For this review, use the dimensioned drawing (mm, ordinates from the lowest corner) and the shaded views. A direction names the side the tool comes from. Coordinates: 2 decimals unless noted, no trailing zeros. Loops run counter-clockwise (first coordinate to the right, second up) from the corner with the lowest first, then second, coordinate; pieces in that order, holes last. Notation, with made-up numbers: M 88,72 L 109,72 A29 cw 109,107 Z; hole C 22,23.5 d2. An arc over 180 degrees is marked long. Write item = value, one per line.
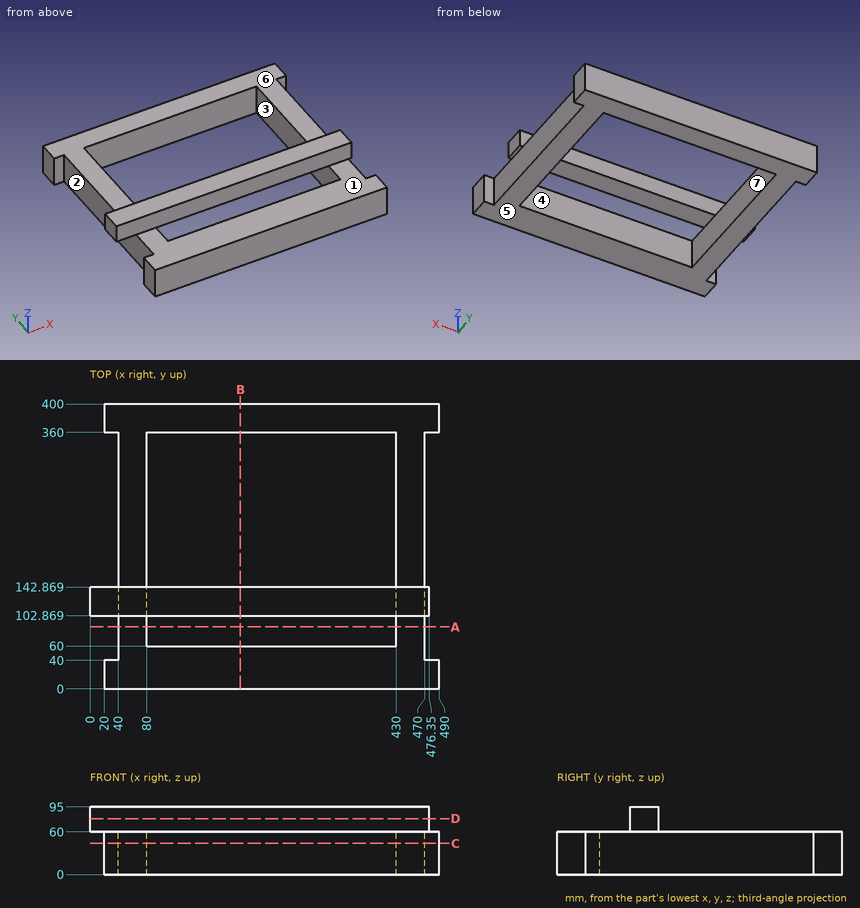
Q1. Draft analysis for pull direction X (two halves, no side actions). For the marked faces 1, 2 and 3, state which applies: +X half, -X half, draft (parallel to the pull), parting line (faces both ways), or undercut.
Solved:
face_1 = draft
face_2 = -X half
face_3 = undercut
Q2. For pin 1 Ø17.5 at (x, z) = (269, 78.5) entering from +Y; pin 2 Ø12 at (y, z) = (372, 24) entering from -X; pin 3 Ø18 at (y, z) = (186, 16) entering from -X, all flat-tipped, find the tip position at first contact; note any pin that passes through.
Solved:
pin_1 = 142.87
pin_2 = 20
pin_3 = 40
Q3. For line 1 along X through (y, z) = (258, 52.5); line 2 along Y through (x, z) = (339, 40.5); line 3 along Z through (x, y) = (30.5, 19), list the stretches that pass through material, from the lowest coordinate up.
Solved:
line_1 = 40 to 80, 430 to 470
line_2 = 0 to 60, 360 to 400
line_3 = 0 to 60
Q4. Add section B-B (x = 211). Write out the cut boundary in (y, z).
Solved:
outline = M 0,0 L 60,0 L 60,60 L 0,60 Z; M 102.87,60 L 142.87,60 L 142.87,95 L 102.87,95 Z; M 360,0 L 400,0 L 400,60 L 360,60 Z
Q5. Machinability: for the marked faces 4, 5, 6 and 7, which of the approach directions +Z, -Z, +X, -X, +Y, -Y give a long, thin tool a straight path to every point of the face, cutting with its end or side? Answer none if there is none.
Solved:
face_4 = +Z, -Z
face_5 = -Z, +X, -X, +Y, -Y
face_6 = +Z, +X, -X, +Y
face_7 = -Z
Q6. Add section A-A (y = 87). Write out the cut boundary in (x, z).
Solved:
outline = M 40,0 L 80,0 L 80,60 L 40,60 Z; M 430,0 L 470,0 L 470,60 L 430,60 Z
Q7. Add section D-D (z = 78.5). Write out the cut boundary in (x, y).
Solved:
outline = M 0,102.87 L 476.35,102.87 L 476.35,142.87 L 0,142.87 Z
Q8. Add section C-C (z = 44). Write out the cut boundary in (x, y).
Solved:
outline = M 20,0 L 490,0 L 490,40 L 470,40 L 470,360 L 490,360 L 490,400 L 20,400 L 20,360 L 40,360 L 40,40 L 20,40 Z; hole M 80,60 L 430,60 L 430,360 L 80,360 Z
